For this review, use the dimensioned drawing (mm, ordinates from the lowest corner) and the shaded views. A direction names the side the tool comes from. Round coordinates to 2 decimals unless told otherwise and drop trailing zeros. Write each loop counter-clockwise with the first axis right and the second up, starting at its lowest first coordinate (ties: lowest second). Pieces come first, ordered by that corner, then holes.
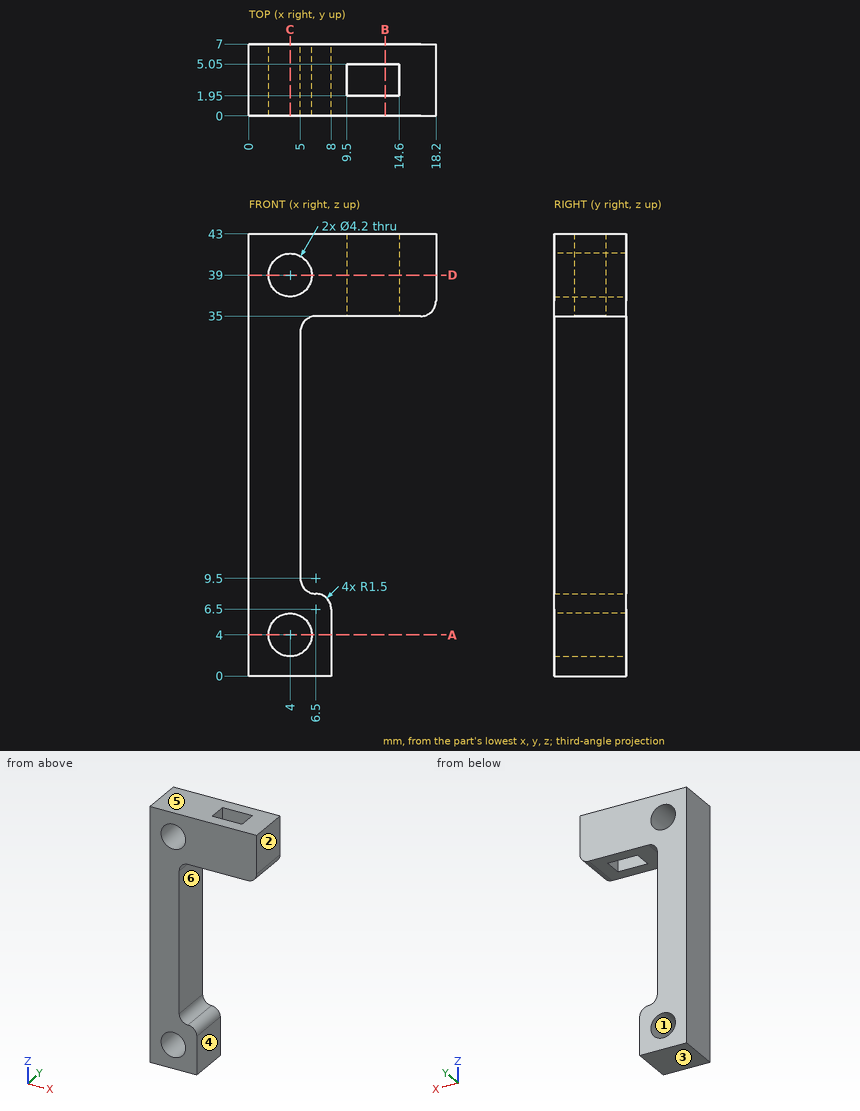
(1) We need section B-B, the plane x = 13.25. Give the boundary of the cut face in (y, z).
Geometry check:
outline: (0, 35) - (1.95, 35) - (1.95, 43) - (0, 43) - close; (5.05, 35) - (7, 35) - (7, 43) - (5.05, 43) - close
(2) For the marked faces 4, 5 and 6, list the 3-axis set-ups (+Z, -Z, +X, -X, +Y, -Y) from which the entire face can be reached by the end or side of a thin tool; tool diameter is ignored.
Geometry check:
face 4: -Z, +X, +Y, -Y
face 5: +Z, +X, -X, +Y, -Y
face 6: +X, +Y, -Y
(3) We need section A-A, the plane z = 4. Give the boundary of the cut face in (x, y).
Geometry check:
outline: (0, 0) - (1.9, 0) - (1.9, 7) - (0, 7) - close; (6.1, 0) - (8, 0) - (8, 7) - (6.1, 7) - close
(4) Mouldability with a two-part tool opening along Z and no side actions: class the marked faces 1, 2 and 3 as pulls with the +Z half, pulls with the -Z half, needs draft (parallel to the pull), parting line crosses it, or undercut.
Geometry check:
face 1: undercut
face 2: needs draft
face 3: pulls with the -Z half
(5) We need section D-D, the plane z = 39. Give the boundary of the cut face in (x, y), and give its area (3 significant figures).
Geometry check:
outline: (0, 0) - (1.9, 0) - (1.9, 7) - (0, 7) - close; (6.1, 0) - (18.2, 0) - (18.2, 7) - (6.1, 7) - close; hole (9.5, 1.95) - (14.6, 1.95) - (14.6, 5.05) - (9.5, 5.05) - close
area: 82.2 mm2
(6) We need section C-C, the plane x = 4. Give the boundary of the cut face in (y, z).
Geometry check:
outline: (0, 0) - (7, 0) - (7, 1.9) - (0, 1.9) - close; (0, 6.1) - (7, 6.1) - (7, 36.9) - (0, 36.9) - close; (0, 41.1) - (7, 41.1) - (7, 43) - (0, 43) - close
(7) For pin 1 Ø3.5 at (y, z) = (2, 25.5) entering from +X; pin 2 Ø2 at (y, z) = (3, 2) entering from +X; pin 3 Ø4 at (x, y) = (13.5, 4) entering from -Z, all flat-tipped, find the tip position at first contact; note any pin that passes through.
Geometry check:
pin 1: stops at x = 5
pin 2: stops at x = 8
pin 3: stops at z = 35
(8) For line 1 along X through (y, z) = (3.75, 39); line 2 along Y through (x, z) = (11.5, 38); line 3 along X through (y, z) = (5, 4), list the stretches that pass through material, from the lowest coordinate up.
Geometry check:
line 1: x = 0 to 1.9, 6.1 to 9.5, 14.6 to 18.2
line 2: y = 0 to 1.95, 5.05 to 7
line 3: x = 0 to 1.9, 6.1 to 8
